```python
from build123d import *

# Parameters (mm, degrees)
SKETCH_1_W      = 100
SKETCH_1_H      = 25
EXTRUDE_1_DEPTH = 38
FILLET_1_R      = 10
FILLET_2_R      = 30
FILLET_3_R      = 10


with BuildPart() as part:
    # 草图1 → 凸台-拉伸1 (new body)
    with BuildSketch(Plane.XY):
        with BuildLine():
            Line((0, 23.5), (0, 25))
            Line((0, 25), (0, 48.210201589))
            Line((0, 48.210201589), (0, 50))
            Line((0, 50), (-50, 50))
            Line((-50, 50), (-50, 0))
            Line((-50, 0), (-23.5, 0))
            ThreePointArc((-23.5, 0), (-16.617009358, 16.617009358), (0, 23.5))
        make_face()
        with BuildLine():
            Line((50, 0), (23.5, 0))
            ThreePointArc((23.5, 0), (16.617009358, -16.617009358), (0, -23.5))
            Line((0, -23.5), (0, -25))
            Line((0, -25), (50, -25))
            Line((50, -25), (50, 0))
        make_face()
        with BuildLine():
            Line((50, 25), (0, 25))
            Line((0, 25), (0, 23.5))
            ThreePointArc((0, 23.5), (16.617009358, 16.617009358), (23.5, 0))
            Line((23.5, 0), (50, 0))
            Line((50, 0), (50, 25))
        make_face()
        Polygon((0, 48.210201589), (0, 25), (50, 25), (50, 50), (0, 50), align=None)
        with Locations((100, 12.5)):
            Rectangle(SKETCH_1_W, SKETCH_1_H)
        with Locations((100, -12.5)):
            Rectangle(SKETCH_1_W, SKETCH_1_H)
        with BuildLine():
            ThreePointArc((0, -23.5), (-16.617009358, -16.617009358), (-23.5, 0))
            Line((-23.5, 0), (-50, 0))
            Line((-50, 0), (-50, -50))
            Line((-50, -50), (50, -50))
            Line((50, -50), (50, -25))
            Line((50, -25), (0, -25))
            Line((0, -25), (0, -23.5))
        make_face()
    extrude(amount=EXTRUDE_1_DEPTH)

    # 圆角1
    fillet_1_edges = [part.edges().sort_by_distance(p)[0] for p in [
        (50, -50, 19),
        (-50, -50, 19),
        (-50, 50, 19),
        (50, 50, 19),
    ]]
    fillet(fillet_1_edges, radius=FILLET_1_R)

    # 圆角2
    fillet_2_edges = [part.edges().sort_by_distance(p)[0] for p in [
        (150, 0, 38),
    ]]
    fillet(fillet_2_edges, radius=FILLET_2_R)

    # 圆角3
    fillet_3_edges = [part.edges().sort_by_distance(p)[0] for p in [
        (85, 25, 38),
        (50, 32.5, 38),
        (0, 50, 38),
        (-50, 0, 38),
        (0, -50, 38),
        (50, -32.5, 38),
        (-47.071067812, 47.071067812, 38),
        (-47.071067812, -47.071067812, 38),
        (85, -25, 38),
        (47.071067812, -47.071067812, 38),
        (47.071067812, 47.071067812, 38),
        (150, 25, 4),
        (141.213203436, 25, 29.213203436),
        (150, -25, 4),
        (141.213203436, -25, 29.213203436),
    ]]
    fillet(fillet_3_edges, radius=FILLET_3_R)


solid = part.part
```
Input: part model. Units: mm. Frame: model coordinates. A direction names the side the tool comes from. Round coordinates to 2 decimals unless told otherwise and drop trailing zeros. Loops run counter-clockwise (first coordinate to the right, second up) from the corner with the lowest first, then second, coordinate; pieces in that order, holes last. Notation, with made-up numbers: (-10.75, 36) -> (16.25, 36) arc R18 ccw to (16.25, 68) -> close; hole circle Ø5 at (26.5, 20). An arc over 180 degrees is marked (long way). Write each question's results on one line, items separated by ' | '.
1. First-contact query: P1, Ø8.5, axis at x = 85.5, z = 16, coming from the -Y side; P2, Ø16.5, axis at y = 30, z = 15, coming from the +X side; P3, Ø12, axis at y = -3.5, z = 27, coming from the +X side. Flat tips, straight axial feed; report the tip coordinate or a pass-through.
Geometry results:
P1: y = -25 | P2: x = 146.69 | P3: x = 147.04
2. Section C-C (x = 117). Return loops of the section in (y, z).
Geometry results:
outline: (-25, 0) -> (25, 0) -> (25, 28) arc R10 ccw to (15, 38) -> (-15, 38) arc R10 ccw to (-25, 28) -> close
3. Section D-D (x = -7). Return loops of the section in (y, z), and give its area (3 significant figures).
Geometry results:
outline: (-50, 0) -> (-22.43, 0) -> (-22.43, 38) -> (-40, 38) arc R10 ccw to (-50, 28) -> close; (22.43, 0) -> (50, 0) -> (50, 28) arc R10 ccw to (40, 38) -> (22.43, 38) -> close | area: 2,050 mm2
4. Section A-A (y = 17.5). Return loops of the section in (x, z).
Geometry results:
outline: (-50, 0) -> (-15.68, 0) -> (-15.68, 38) -> (-40, 38) arc R10 ccw to (-50, 28) -> close; (15.68, 0) -> (149.68, 0) -> (149.68, 8) arc R29.68 ccw to (120, 37.68) -> (42.5, 37.68) arc R10 ccw to (40, 38) -> (15.68, 38) -> close
5. Set-up query: faces 1 (the face through (80.56, 21.99, 35.15)), 2 (the face through (50, 32, 14)), 3 (the face through (94, -25, 14)). Return all of +Z, -Z, +X, -X, +Y, -Y with unobstructed straight access to the full face (end or side cutting, diameter ignored); none if empty.
Geometry results:
face 1: +Z, +X, +Y | face 2: +Z, -Z, +X, +Y | face 3: +Z, -Z, +X, -Y
6. Section B-B (z = 2.5). Return loops of the section in (x, y).
Geometry results:
outline: (-50, -40) arc R10 ccw to (-40, -50) -> (40, -50) arc R10 ccw to (50, -40) -> (50, -25) -> (140, -25) arc R10 ccw to (150, -15) -> (150, 15) arc R10 ccw to (140, 25) -> (50, 25) -> (50, 40) arc R10 ccw to (40, 50) -> (-40, 50) arc R10 ccw to (-50, 40) -> close; hole circle Ø47 at (0, 0)
7. Ray query, line 1 (Y direction, x = 1, z = 28.5); line 2 (X direction, y = 31.5, z = 9); line 3 (Y direction, x = 58.5, z = 25). Return the intervals inside material, ascending. Write a range as from..to.
Geometry results:
line 1: -49.99..-23.48, 23.48..49.99 | line 2: -50..50 | line 3: -25..25
